Could you check a few things on this model? Use its own coordinates, in mm. A direction names the side the tool comes from. Give positions to 0.01 mm unless a question says otherwise; leave off trailing zeros. Order: outer loops, then holes, each group sorted by start corner. A loop starts at its lowest first (then second) coordinate and runs counter-clockwise, first axis right, second up. Notation, with made-up numbers: (-4, -5.5) -> (29, -5.5) arc R16 ccw to (29, 11.5) -> close; hole circle Ø9 at (-2.75, 51). An arc over 180 degrees is marked (long way). One line per item, written item: value.
Autodesk Inventor part; units mm, degrees
ref_plane "YZ Plane" through (0, 0, 0) normal (1, 0, 0) x (0, 1, 0)
ref_plane "XZ Plane" through (0, 0, 0) normal (0, 1, 0) x (-1, 0, 0)
ref_plane "XY Plane" through (0, 0, 0) normal (0, 0, 1) x (1, 0, 0)
sketch "Sketch2" plane through (0, 0, 0) normal (0, 0, 1) x (1, 0, 0)
  line L0 (0, 0) -> (60, 0)
  line L1 (60, 0) -> (60, 40)
  line L2 (60, 40) -> (0, 40)
  line L3 (0, 40) -> (0, 0)
  dimension "d11" = 60
  dimension "d12" = 40
extrude "Extrusion1" add sketch "Sketch2" along normal blind 45
shell "Shell1" thickness 5 removed faces 2 at (20, 26.6667, 45) at (60, 13.3333, 30)
sketch "Sketch4" plane through (0, 0, 45) normal (0, 0, 1) x (1, 0, 0)
  line L0 (5, 35) -> (5, 5)
  circle A0 centre (2.4749, 37.4236) radius 2
  circle A1 centre (2.4749, 2.5764) radius 2
  point P0 (0, 0)
  dimension "d20" = 4
  dimension "d21" = 4
hole "Hole2" at (2.4749, 37.4236, 45) direction (0, 0, -1) diameter 3 depth 9 tip angle 118
sketch "Sketch6" plane through (0, 0, 45) normal (0, 0, 1) x (1, 0, 0)
  line L0 (5, 35) -> (5, 5)
  circle A0 centre (2.5251, 2.5251) radius 2
  point P0 (0, 0)
  dimension "d37" = 4
hole "Hole3" at (2.5251, 2.5251, 45) direction (0, 0, -1) diameter 3 depth 9 tip angle 118
sketch "Sketch7" plane through (60, 0, 0) normal (1, 0, 0) x (0, 0, -1)
  line L0 (-5, 35) -> (-45, 35)
  circle A0 centre (-2.5251, 37.4749) radius 2
  point P0 (0, 0)
  dimension "d46" = 4
hole "Hole4" at (60, 37.4749, 2.5251) direction (-1, 0, 0) diameter 3 depth 9 tip angle 118
sketch "Sketch8" plane through (60, 0, 0) normal (1, 0, 0) x (0, 0, -1)
  line L0 (-5, 35) -> (-5, 5)
  circle A0 centre (-2.5251, 2.5251) radius 2
  point P0 (0, 0)
  dimension "d55" = 4
hole "Hole5" at (60, 2.5251, 2.5251) direction (-1, 0, 0) diameter 3 depth 9 tip angle 118
sketch "Sketch11" plane through (0, 0, 45) normal (0, 0, 1) x (1, 0, 0)
  line L0 (60, 35) -> (5, 35)
  line L1 (60, 38.9749) -> (60, 35.9749)
  line L2 (5, 35) -> (60, 35)
  line L3 (60, 35) -> (60, 38)
  line L4 (60, 38) -> (5, 38)
  line L5 (5, 38) -> (5, 35)
  point P0 (0, 0)
  dimension "d76" = 3
extrude "Extrusion4" cut sketch "Sketch11" against normal blind 40
sketch "Sketch12" plane through (0, 0, 45) normal (0, 0, 1) x (1, 0, 0)
  line L0 (5, 38) -> (5, 5)
  line L1 (60, 4.0251) -> (60, 1.0251)
  line L2 (5, 5) -> (60, 5)
  line L3 (60, 5) -> (60, 2)
  line L4 (60, 2) -> (5, 2)
  line L5 (5, 2) -> (5, 5)
  point P0 (0, 0)
  dimension "d79" = 3
extrude "Extrusion5" cut sketch "Sketch12" against normal blind 40
sketch "Sketch13" plane through (0, 0, 45) normal (0, 0, 1) x (1, 0, 0)
  line L0 (5, 38) -> (60, 38)
  line L1 (5, 38) -> (5, 35)
  line L2 (5, 2) -> (5, 38)
  line L3 (5, 35) -> (2, 35)
  line L4 (2, 35) -> (2, 5)
  line L5 (2, 5) -> (5, 5)
  line L6 (5, 5) -> (5, 35)
  point P0 (0, 0)
  dimension "d82" = 3
  dimension "d83" = 3
  dimension "d84" = 30
extrude "Extrusion6" cut sketch "Sketch13" against normal blind 40
sketch "Sketch14" plane through (60, 0, 0) normal (1, 0, 0) x (0, 0, -1)
  line L0 (-5, 38) -> (-5, 2)
  line L1 (-5, 38) -> (-5, 35)
  line L2 (-5, 35) -> (-2, 35)
  line L3 (-2, 35) -> (-2, 5)
  line L4 (-2, 5) -> (-5, 5)
  line L5 (-5, 5) -> (-5, 35)
  point P0 (0, 0)
  dimension "d87" = 3
  dimension "d88" = 3
  dimension "d89" = 30
extrude "Extrusion7" cut sketch "Sketch14" against normal blind 58
sketch "Sketch18" plane through (5, 38, 45) normal (0, -1, 0) x (1, 0, 0)
  line L0 (0, -40) -> (55, -40)
  line L1 (55, -40) -> (55, -25)
  line L2 (55, 0) -> (55, -40)
  line L3 (55, -25) -> (49, -25)
  circle A0 centre (48.7205, -25) radius 1.5
  point P0 (-5, -45)
  dimension "d108" = 15
  dimension "d109" = 6
  dimension "d110" = 3
extrude "Extrusion10" cut sketch "Sketch18" against normal blind 2
sketch "Sketch19" plane through (0, 0, 0) normal (0, 0, -1) x (-1, 0, 0)
  line L0 (0, 0) -> (0, 40)
  line L1 (0, 40) -> (-30, 40)
  line L2 (-2, 40) -> (-60, 40)
  line L3 (-30, 40) -> (-17.5, 40)
  line L4 (-17.5, 40) -> (-42.5, 40)
  line L5 (-42.5, 40) -> (-42.5, 35)
  line L6 (-42.5, 35) -> (-17.5, 35)
  line L7 (-17.5, 35) -> (-17.5, 40)
  dimension "d113" = 40
  dimension "d114" = 30
  dimension "d115" = 12.5
  dimension "d116" = 25
  dimension "d117" = 5
extrude "Extrusion11" add sketch "Sketch19" along normal blind 7
sketch "Sketch20" plane through (0, 40, 45) normal (0, 1, 0) x (1, 0, 0)
  line L0 (42.5, 45) -> (40, 45)
  line L1 (17.5, 45) -> (42.5, 45)
  line L2 (40, 45) -> (20, 45)
  line L3 (20, 45) -> (20, 49.5)
  line L4 (20, 49.5) -> (40, 49.5)
  line L5 (40, 49.5) -> (40, 45)
  point P0 (0, 45)
  dimension "d120" = 2.5
  dimension "d121" = 20
  dimension "d122" = 4.5
extrude "Extrusion12" cut sketch "Sketch20" against normal blind 5
fillet "Fillet3" radius 1 9 edges at (51.25, 40, 0) (42.5, 40, -3.5) (30, 40, -7) (17.5, 40, -3.5) (8.75, 40, 0) (0, 40, 22.5) (0, 20, 0) (30, 0, 0) (0, 0, 22.5)
fillet "Fillet4" radius 2 7 edges at (42.2071, 39.7071, -6.7071) (42.5, 37, -7) (30, 35, -7) (17.5, 37, -7) (17.7929, 39.7071, -6.7071) (42.5, 35, -3.5) (17.5, 35, -3.5)
sketch "Sketch21" plane through (1, 40, 45) normal (0, 1, 0) x (1, 0, 0)
  point P0 (-1, 45)
properties material "ABS Plastic"
1) Suppose I cut it at D-D, the plane x = 48. Write out the boundary of the cut face in (y, z).
Answer below:
outline: (0, 1) arc R1 ccw to (1, 0) -> (39, 0) arc R1 ccw to (40, 1) -> (40, 45) -> (38, 45) -> (38, 5) -> (35, 5) -> (35, 2) -> (5, 2) -> (5, 5) -> (2, 5) -> (2, 45) -> (0, 45) -> close
2) If I drill on line 1 along Y through (x, z) = (28, 34.5); line 2 along Y through (x, z) = (3, 21); line 3 along X through (y, z) = (13, 17), over which ranges is the centre line in solid material (lowest first)?
Answer below:
line 1: y = 0 to 2, 38 to 40
line 2: y = 0 to 5, 35 to 40
line 3: x = 0 to 2
3) We'd pull the mould along Y, two halves only. Please class faces 4 (the conical face through (50.26, 2.29, 2.4)), 5 (the flat face through (30, 38, -7)), 6 (the cylindrical face through (41.9, 35.57, -2.46)): +Y half, -Y half, draft (parallel to the pull), parting line (faces both ways), or undercut.
Answer below:
face 4: undercut
face 5: draft
face 6: -Y half
4) For faces 1 (the flat face through (32, 4, 5)), 2 (the flat face through (30, 38, -4.5)), 3 (the flat face through (17.5, 38, -2)), which set-ups out of +Z, -Z, +X, -X, +Y, -Y let a thin tool reach every point of the face, with its end or its side?
Answer below:
face 1: +Z, +X
face 2: +Y, -Y
face 3: -Z, -X, +Y, -Y
5) Suppose I cut it at B-B, the plane z = 20. Write out the boundary of the cut face in (x, y).
Answer below:
outline: (0, 1) arc R1 ccw to (1, 0) -> (60, 0) -> (60, 2) -> (5, 2) -> (5, 5) -> (2, 5) -> (2, 35) -> (5, 35) -> (5, 38) -> (52.22, 38) -> (52.22, 40) -> (1, 40) arc R1 ccw to (0, 39) -> close; (55.22, 38) -> (60, 38) -> (60, 40) -> (55.22, 40) -> close
6) Suppose I cut it at C-C, the plane y = 21.5. Write out the boundary of the cut face in (x, z).
Answer below:
outline: (0, 1) arc R1 ccw to (1, 0) -> (60, 0) -> (60, 2) -> (2, 2) -> (2, 45) -> (0, 45) -> close
7) Suppose I cut it at A-A, the plane x = 34. Write out the boundary of the cut face in (y, z), then the cut area to 3 significant figures.
Answer below:
outline: (0, 1) arc R1 ccw to (1, 0) -> (40, 0) -> (40, 45) -> (38, 45) -> (38, 5) -> (35, 5) -> (35, 2) -> (5, 2) -> (5, 5) -> (2, 5) -> (2, 45) -> (0, 45) -> close; (35, -5) arc R2 ccw to (37, -7) -> (39, -7) arc R1 ccw to (40, -6) -> (40, -4.5) -> (35, -4.5) -> close
area: 281 mm2
8) For P1, Ø6, axis at x = 51.5, y = 15.5, coming from the +Z side; P2, Ø0.9, axis at y = 4, z = 18.5, coming from the +X side; P3, Ø5, axis at x = 26, y = 8.5, coming from the -Z side, each with a flat end and sliding along its axis, tell me the tip position at first contact or that it passes through.
Answer below:
P1: stops at z = 2
P2: stops at x = 5
P3: stops at z = 0
